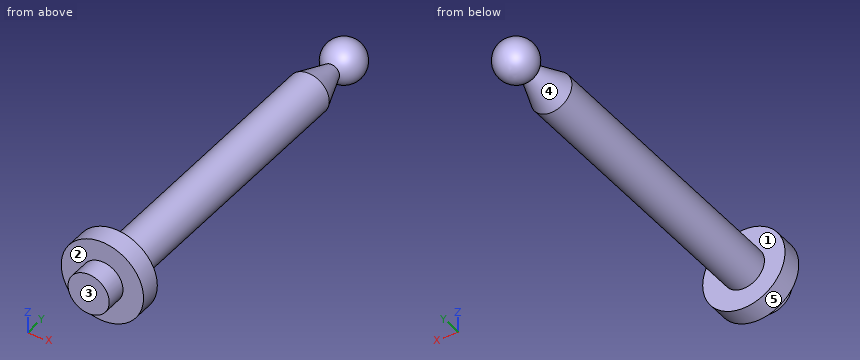
from build123d import *

# Parameters (mm, degrees)
SKETCH1_R           = 5
BOSS_EXTRUDE1_DEPTH = 5
SKETCH2_R           = 10
BOSS_EXTRUDE2_DEPTH = 5
SKETCH3_R           = 5
BOSS_EXTRUDE3_DEPTH = 70


with BuildPart() as part:
    # Sketch1 → Boss-Extrude1 (new body)
    with BuildSketch(Plane(origin=(0, 0, 0), x_dir=(1, 0, 0), z_dir=(0, 1, 0))):
        Circle(SKETCH1_R)
    extrude(amount=BOSS_EXTRUDE1_DEPTH)

    # Sketch2 → Boss-Extrude2 (add)
    with BuildSketch(Plane(origin=(0, 5, 0), x_dir=(1, 0, 0), z_dir=(0, 1, 0))):
        Circle(SKETCH2_R)
    extrude(amount=BOSS_EXTRUDE2_DEPTH)

    # Sketch3 → Boss-Extrude3 (add)
    with BuildSketch(Plane(origin=(0, 10, 0), x_dir=(1, 0, 0), z_dir=(0, 1, 0))):
        Circle(SKETCH3_R)
    extrude(amount=BOSS_EXTRUDE3_DEPTH)

    # Sketch4 → Revolve1 (revolve)
    with BuildSketch(Plane(origin=(0, 0, 0), x_dir=(0, 0, -1), z_dir=(1, 0, 0))):
        with BuildLine():
            Line((5, 80), (2, 88.242432258))
            ThreePointArc((2, 88.242432258), (4.894531565, 93.846556172), (0, 97.825007953))
            Line((0, 97.825007953), (0, 80))
            Line((0, 80), (5, 80))
        make_face()
    revolve(axis=Axis((0, 97.825007953, 0), (0, -1, 0)))


solid = part.part
The listing builds one solid part. Answer for the finished solid, in the listing's coordinates (mm). Face numbers are marked on the shaded views. A direction names the side the tool comes from. Coordinates: 2 decimals unless noted, no trailing zeros. Order: outer loops, then holes, each group sorted by start corner. A loop starts at its lowest first (then second) coordinate and runs counter-clockwise, first axis right, second up. Notation, with made-up numbers: (31, 86) -> (77, 86) arc R12 ccw to (77, 106) -> close; hole circle Ø4 at (34.5, 60.25). An arc over 180 degrees is marked (long way). Answer in a Markdown table with one row per item. Add a question column.
Item 1: Each of these flat-tipped pins is pushed along its axis until it touches: P1, Ø5, axis at y = 26, z = -6.5, coming from the +X side; P2, Ø1.5, axis at x = 4.5, z = 1.5, coming from the +Y side; P3, Ø5, axis at x = 6.5, y = 69, coming from the +Z side; P4, Ø6, axis at x = 0.5, z = 2, coming from the +Y side (3 decimals). Where does it stop, or does it pass through?
Item 2: Find section C-C (y = 49.5). Write down the section's boundary in (x, z), then the cut area to 3 significant figures.
Item 3: Which of the six approach directions +Z, -Z, +X, -X, +Y, -Y give full straight-line access (tool end or side, diameter ignored) to the marked faces 1, 2, 3, 4 and 5?
Item 4: Find section D-D (z = -8). Write down the section's boundary in (x, y).
Item 5: Find section A-A (z = 0). Write down the section's boundary in (x, y) (3 decimals).
Item 6: Find the intervals of material crossed by L1, parallel to X at y = 35.5, z = 0; L2, parallel to Y at x = 4.25, z = -4; L3, parallel to Y at x = -3.5, z = -3, in increasing order. Write a range as from..to.
Item 7: Find section B-B (x = 0). Write down the section's boundary in (y, z) (3 decimals).
Result set:
| question | item | result |
|---|---|---|
| 1 | P1 | stops at x = 3 |
| 1 | P2 | stops at y = 95.83 |
| 1 | P3 | stops at z = 3 |
| 1 | P4 | stops at y = 97.825 |
| 2 | outline | circle Ø10 at (0, 0) |
| 2 | area | 78.5 mm² |
| 3 | face 1 | +Y |
| 3 | face 2 | -Y |
| 3 | face 3 | +Z, -Z, +X, -X, -Y |
| 3 | face 4 | none |
| 3 | face 5 | +Y, -Y |
| 4 | outline | (-6, 5) -> (6, 5) -> (6, 10) -> (-6, 10) -> close |
| 5 | outline | (-10, 5) -> (-5, 5) -> (-5, 0) -> (5, 0) -> (5, 5) -> (10, 5) -> (10, 10) -> (5, 10) -> (5, 80) -> (2, 88.242) arc R5 ccw (long way) to (-2, 88.242) -> (-5, 80) -> (-5, 10) -> (-10, 10) -> close |
| 6 | L1 | x = -5..5 |
| 6 | L2 | y = 5..10 |
| 6 | L3 | y = 0..81.07, 90.89..94.76 |
| 7 | outline | (0, -5) -> (5, -5) -> (5, -10) -> (10, -10) -> (10, -5) -> (80, -5) -> (88.242, -2) arc R5 ccw (long way) to (88.242, 2) -> (80, 5) -> (10, 5) -> (10, 10) -> (5, 10) -> (5, 5) -> (0, 5) -> close |
